from build123d import *

# Parameters (mm, degrees)
SKETCH1_W           = 748
SKETCH1_H           = 180
SKETCH1_R           = 2.5
SKETCH1_R_2         = 6
SKETCH1_W_2         = 100
SKETCH1_H_2         = 95
BOSS_EXTRUDE1_DEPTH = 4


with BuildPart() as part:
    # Sketch1 → Boss-Extrude1 (new body)
    with BuildSketch(Plane(origin=(0, 0, 0), x_dir=(1, 0, 0), z_dir=(0, 1, 0))):
        Rectangle(SKETCH1_W, SKETCH1_H)
        with Locations((-344, 80)):
            Circle(SKETCH1_R, mode=Mode.SUBTRACT)
        with Locations((0, 80)):
            Circle(SKETCH1_R, mode=Mode.SUBTRACT)
        with Locations((344, 80)):
            Circle(SKETCH1_R, mode=Mode.SUBTRACT)
        with Locations((-344, -80)):
            Circle(SKETCH1_R, mode=Mode.SUBTRACT)
        with Locations((0, -80)):
            Circle(SKETCH1_R, mode=Mode.SUBTRACT)
        with Locations((344, -80)):
            Circle(SKETCH1_R, mode=Mode.SUBTRACT)
        with Locations((-360, 80)):
            Circle(SKETCH1_R_2, mode=Mode.SUBTRACT)
        with Locations((-360, -80)):
            Circle(SKETCH1_R_2, mode=Mode.SUBTRACT)
        with Locations((360, -80)):
            Circle(SKETCH1_R_2, mode=Mode.SUBTRACT)
        with Locations((360, 80)):
            Circle(SKETCH1_R_2, mode=Mode.SUBTRACT)
        with Locations((-214, -17.5)):
            Rectangle(SKETCH1_W_2, SKETCH1_H_2, mode=Mode.SUBTRACT)
    extrude(amount=BOSS_EXTRUDE1_DEPTH)


solid = part.part
Here's how the part is built. I have some questions about the finished solid (model axes, mm). Give positions to 0.01 mm unless a question says otherwise; leave off trailing zeros. Answer as a JSON object with one key per item and string values. Group by question number.
Item 1: Imagine slicing it at A-A on y = 2. Give the number of separate pieces and of enclosed holes in the cut face, then the cut area to 3 significant figures.
Item 2: Will this pin go through, and if not, where does the flat tip stop? pin 1 (11 mm diameter, centred on x = -360, z = 80, fed in from -Y).
Item 3: I need wall thicknesses on L1, parallel to X at y = 1, z = -80; L2, parallel to Z at x = 344, y = 1.7; L3, parallel to Z at x = -360, y = 2.1. Which ranges of each line are inside material? Lowest first, please.
Item 4: Thinking about a two-plate mould opening in Z: for faces 1 (the cylindrical face through (365.723, 1.972, 78.198)), 2 (the flat face through (-5, 0, -1)), which applies, pulls with the +Z half, pulls with the -Z half, needs draft (parallel to the pull), parting line crosses it, or undercut?
Answer list:
{
 "1": {"separate pieces": "1", "enclosed holes": "11", "area": "125,000 mm2"},
 "2": {"pin 1": "passes through"},
 "3": {"L1": "x = -374 to -366, -354 to -346.5, -341.5 to -2.5, 2.5 to 341.5, 346.5 to 354, 366 to 374", "L2": "z = -90 to -82.5, -77.5 to 77.5, 82.5 to 90", "L3": "z = -90 to -86, -74 to 74, 86 to 90"},
 "4": {"face 1": "undercut", "face 2": "needs draft"}
}
